CAD build for the part. Positions are in the model's coordinates, mm. A direction names the side the tool comes from. Round coordinates to 2 decimals unless told otherwise and drop trailing zeros. Order: outer loops, then holes, each group sorted by start corner. A loop starts at its lowest first (then second) coordinate and runs counter-clockwise, first axis right, second up. Notation, with made-up numbers: M 11.25,14 L 21.25,14 A37 cw 21.25,50 Z; hole C 48,68 d5. An arc over 180 degrees is marked long. Put each result on its own line as item: value.
```python
from build123d import *

# Parameters (mm, degrees)
SKETCH1_W                = 9
SKETCH1_H                = 2
BOSS_EXTRUDE1_DEPTH      = 15
CUT_EXTRUDE1_START       = -31
SKETCH2_W                = 8
SKETCH2_H                = 0.6
CUT_EXTRUDE1_DEPTH       = 32
SKETCH3_W                = 7.634272068
SKETCH3_H                = 0.75
CUT_EXTRUDE2_DEPTH       = 0.2
LPATTERN1_COUNT          = 19
LPATTERN1_PITCH          = 1.5
MIRROR2_COPY_1_SKETCH_W  = 7.634272068
MIRROR2_COPY_1_SKETCH_H  = 0.75
MIRROR2_COPY_1_DEPTH     = 0.2
MIRROR2_COPY_2_SKETCH_W  = 7.634272068
MIRROR2_COPY_2_SKETCH_H  = 0.75
MIRROR2_COPY_2_DEPTH     = 0.2
MIRROR2_COPY_3_SKETCH_W  = 7.634272068
MIRROR2_COPY_3_SKETCH_H  = 0.75
MIRROR2_COPY_3_DEPTH     = 0.2
MIRROR2_COPY_4_SKETCH_W  = 7.634272068
MIRROR2_COPY_4_SKETCH_H  = 0.75
MIRROR2_COPY_4_DEPTH     = 0.2
MIRROR2_COPY_5_SKETCH_W  = 7.634272068
MIRROR2_COPY_5_SKETCH_H  = 0.75
MIRROR2_COPY_5_DEPTH     = 0.2
MIRROR2_COPY_6_SKETCH_W  = 7.634272068
MIRROR2_COPY_6_SKETCH_H  = 0.75
MIRROR2_COPY_6_DEPTH     = 0.2
MIRROR2_COPY_7_SKETCH_W  = 7.634272068
MIRROR2_COPY_7_SKETCH_H  = 0.75
MIRROR2_COPY_7_DEPTH     = 0.2
MIRROR2_COPY_8_SKETCH_W  = 7.634272068
MIRROR2_COPY_8_SKETCH_H  = 0.75
MIRROR2_COPY_8_DEPTH     = 0.2
MIRROR2_COPY_9_SKETCH_W  = 7.634272068
MIRROR2_COPY_9_SKETCH_H  = 0.75
MIRROR2_COPY_9_DEPTH     = 0.2
MIRROR2_COPY_10_SKETCH_W = 7.634272068
MIRROR2_COPY_10_SKETCH_H = 0.75
MIRROR2_COPY_10_DEPTH    = 0.2
MIRROR2_COPY_11_SKETCH_W = 7.634272068
MIRROR2_COPY_11_SKETCH_H = 0.75
MIRROR2_COPY_11_DEPTH    = 0.2
MIRROR2_COPY_12_SKETCH_W = 7.634272068
MIRROR2_COPY_12_SKETCH_H = 0.75
MIRROR2_COPY_12_DEPTH    = 0.2
MIRROR2_COPY_13_SKETCH_W = 7.634272068
MIRROR2_COPY_13_SKETCH_H = 0.75
MIRROR2_COPY_13_DEPTH    = 0.2
MIRROR2_COPY_14_SKETCH_W = 7.634272068
MIRROR2_COPY_14_SKETCH_H = 0.75
MIRROR2_COPY_14_DEPTH    = 0.2
MIRROR2_COPY_15_SKETCH_W = 7.634272068
MIRROR2_COPY_15_SKETCH_H = 0.75
MIRROR2_COPY_15_DEPTH    = 0.2
MIRROR2_COPY_16_SKETCH_W = 7.634272068
MIRROR2_COPY_16_SKETCH_H = 0.75
MIRROR2_COPY_16_DEPTH    = 0.2
MIRROR2_COPY_17_SKETCH_W = 7.634272068
MIRROR2_COPY_17_SKETCH_H = 0.75
MIRROR2_COPY_17_DEPTH    = 0.2
MIRROR2_COPY_18_SKETCH_W = 7.634272068
MIRROR2_COPY_18_SKETCH_H = 0.75
MIRROR2_COPY_18_DEPTH    = 0.2


with BuildPart() as part:
    # Sketch1 → Boss-Extrude1 (new body, symmetric)
    with BuildSketch(Plane(origin=(0, 0, 0), x_dir=(1, 0, 0), z_dir=(0, 1, 0))):
        Rectangle(SKETCH1_W, SKETCH1_H)
    extrude(amount=BOSS_EXTRUDE1_DEPTH, both=True)

    # Sketch2 → Cut-Extrude1 (cut)
    with BuildSketch(Plane(origin=(0, 15, 0), x_dir=(1, 0, 0), z_dir=(0, 1, 0)).offset(CUT_EXTRUDE1_START)):
        with Locations((0, 0.5)):
            Rectangle(SKETCH2_W, SKETCH2_H)
    cut_extrude1 = extrude(amount=CUT_EXTRUDE1_DEPTH, mode=Mode.SUBTRACT)

    # Mirror1: Cut-Extrude1 across plane
    add(cut_extrude1.mirror(Plane.XY), mode=Mode.SUBTRACT)

    # Sketch3 → Cut-Extrude2 (cut)
    with BuildSketch(Plane.XY.offset(1)):
        with Locations((0, 13.875)):
            Rectangle(SKETCH3_W, SKETCH3_H)
    cut_extrude2 = extrude(amount=-CUT_EXTRUDE2_DEPTH, mode=Mode.SUBTRACT)

    # LPattern1: Cut-Extrude2 ×19
    with Locations(*[(0, -i * LPATTERN1_PITCH, 0) for i in range(1, LPATTERN1_COUNT)]):
        add(cut_extrude2, mode=Mode.SUBTRACT)

    # Mirror2: Cut-Extrude2 across plane
    add(cut_extrude2.mirror(Plane.XY), mode=Mode.SUBTRACT)

    # Mirror2 copy 1 sketch → Mirror2 copy 1 (cut)
    with BuildSketch(Plane(origin=(0, -1.5, -1), x_dir=(1, 0, 0), z_dir=(0, 0, -1))):
        with Locations((0, -13.875)):
            Rectangle(MIRROR2_COPY_1_SKETCH_W, MIRROR2_COPY_1_SKETCH_H)
    extrude(amount=-MIRROR2_COPY_1_DEPTH, mode=Mode.SUBTRACT)

    # Mirror2 copy 2 sketch → Mirror2 copy 2 (cut)
    with BuildSketch(Plane(origin=(0, -3, -1), x_dir=(1, 0, 0), z_dir=(0, 0, -1))):
        with Locations((0, -13.875)):
            Rectangle(MIRROR2_COPY_2_SKETCH_W, MIRROR2_COPY_2_SKETCH_H)
    extrude(amount=-MIRROR2_COPY_2_DEPTH, mode=Mode.SUBTRACT)

    # Mirror2 copy 3 sketch → Mirror2 copy 3 (cut)
    with BuildSketch(Plane(origin=(0, -4.5, -1), x_dir=(1, 0, 0), z_dir=(0, 0, -1))):
        with Locations((0, -13.875)):
            Rectangle(MIRROR2_COPY_3_SKETCH_W, MIRROR2_COPY_3_SKETCH_H)
    extrude(amount=-MIRROR2_COPY_3_DEPTH, mode=Mode.SUBTRACT)

    # Mirror2 copy 4 sketch → Mirror2 copy 4 (cut)
    with BuildSketch(Plane(origin=(0, -6, -1), x_dir=(1, 0, 0), z_dir=(0, 0, -1))):
        with Locations((0, -13.875)):
            Rectangle(MIRROR2_COPY_4_SKETCH_W, MIRROR2_COPY_4_SKETCH_H)
    extrude(amount=-MIRROR2_COPY_4_DEPTH, mode=Mode.SUBTRACT)

    # Mirror2 copy 5 sketch → Mirror2 copy 5 (cut)
    with BuildSketch(Plane(origin=(0, -7.5, -1), x_dir=(1, 0, 0), z_dir=(0, 0, -1))):
        with Locations((0, -13.875)):
            Rectangle(MIRROR2_COPY_5_SKETCH_W, MIRROR2_COPY_5_SKETCH_H)
    extrude(amount=-MIRROR2_COPY_5_DEPTH, mode=Mode.SUBTRACT)

    # Mirror2 copy 6 sketch → Mirror2 copy 6 (cut)
    with BuildSketch(Plane(origin=(0, -9, -1), x_dir=(1, 0, 0), z_dir=(0, 0, -1))):
        with Locations((0, -13.875)):
            Rectangle(MIRROR2_COPY_6_SKETCH_W, MIRROR2_COPY_6_SKETCH_H)
    extrude(amount=-MIRROR2_COPY_6_DEPTH, mode=Mode.SUBTRACT)

    # Mirror2 copy 7 sketch → Mirror2 copy 7 (cut)
    with BuildSketch(Plane(origin=(0, -10.5, -1), x_dir=(1, 0, 0), z_dir=(0, 0, -1))):
        with Locations((0, -13.875)):
            Rectangle(MIRROR2_COPY_7_SKETCH_W, MIRROR2_COPY_7_SKETCH_H)
    extrude(amount=-MIRROR2_COPY_7_DEPTH, mode=Mode.SUBTRACT)

    # Mirror2 copy 8 sketch → Mirror2 copy 8 (cut)
    with BuildSketch(Plane(origin=(0, -12, -1), x_dir=(1, 0, 0), z_dir=(0, 0, -1))):
        with Locations((0, -13.875)):
            Rectangle(MIRROR2_COPY_8_SKETCH_W, MIRROR2_COPY_8_SKETCH_H)
    extrude(amount=-MIRROR2_COPY_8_DEPTH, mode=Mode.SUBTRACT)

    # Mirror2 copy 9 sketch → Mirror2 copy 9 (cut)
    with BuildSketch(Plane(origin=(0, -13.5, -1), x_dir=(1, 0, 0), z_dir=(0, 0, -1))):
        with Locations((0, -13.875)):
            Rectangle(MIRROR2_COPY_9_SKETCH_W, MIRROR2_COPY_9_SKETCH_H)
    extrude(amount=-MIRROR2_COPY_9_DEPTH, mode=Mode.SUBTRACT)

    # Mirror2 copy 10 sketch → Mirror2 copy 10 (cut)
    with BuildSketch(Plane(origin=(0, -15, -1), x_dir=(1, 0, 0), z_dir=(0, 0, -1))):
        with Locations((0, -13.875)):
            Rectangle(MIRROR2_COPY_10_SKETCH_W, MIRROR2_COPY_10_SKETCH_H)
    extrude(amount=-MIRROR2_COPY_10_DEPTH, mode=Mode.SUBTRACT)

    # Mirror2 copy 11 sketch → Mirror2 copy 11 (cut)
    with BuildSketch(Plane(origin=(0, -16.5, -1), x_dir=(1, 0, 0), z_dir=(0, 0, -1))):
        with Locations((0, -13.875)):
            Rectangle(MIRROR2_COPY_11_SKETCH_W, MIRROR2_COPY_11_SKETCH_H)
    extrude(amount=-MIRROR2_COPY_11_DEPTH, mode=Mode.SUBTRACT)

    # Mirror2 copy 12 sketch → Mirror2 copy 12 (cut)
    with BuildSketch(Plane(origin=(0, -18, -1), x_dir=(1, 0, 0), z_dir=(0, 0, -1))):
        with Locations((0, -13.875)):
            Rectangle(MIRROR2_COPY_12_SKETCH_W, MIRROR2_COPY_12_SKETCH_H)
    extrude(amount=-MIRROR2_COPY_12_DEPTH, mode=Mode.SUBTRACT)

    # Mirror2 copy 13 sketch → Mirror2 copy 13 (cut)
    with BuildSketch(Plane(origin=(0, -19.5, -1), x_dir=(1, 0, 0), z_dir=(0, 0, -1))):
        with Locations((0, -13.875)):
            Rectangle(MIRROR2_COPY_13_SKETCH_W, MIRROR2_COPY_13_SKETCH_H)
    extrude(amount=-MIRROR2_COPY_13_DEPTH, mode=Mode.SUBTRACT)

    # Mirror2 copy 14 sketch → Mirror2 copy 14 (cut)
    with BuildSketch(Plane(origin=(0, -21, -1), x_dir=(1, 0, 0), z_dir=(0, 0, -1))):
        with Locations((0, -13.875)):
            Rectangle(MIRROR2_COPY_14_SKETCH_W, MIRROR2_COPY_14_SKETCH_H)
    extrude(amount=-MIRROR2_COPY_14_DEPTH, mode=Mode.SUBTRACT)

    # Mirror2 copy 15 sketch → Mirror2 copy 15 (cut)
    with BuildSketch(Plane(origin=(0, -22.5, -1), x_dir=(1, 0, 0), z_dir=(0, 0, -1))):
        with Locations((0, -13.875)):
            Rectangle(MIRROR2_COPY_15_SKETCH_W, MIRROR2_COPY_15_SKETCH_H)
    extrude(amount=-MIRROR2_COPY_15_DEPTH, mode=Mode.SUBTRACT)

    # Mirror2 copy 16 sketch → Mirror2 copy 16 (cut)
    with BuildSketch(Plane(origin=(0, -24, -1), x_dir=(1, 0, 0), z_dir=(0, 0, -1))):
        with Locations((0, -13.875)):
            Rectangle(MIRROR2_COPY_16_SKETCH_W, MIRROR2_COPY_16_SKETCH_H)
    extrude(amount=-MIRROR2_COPY_16_DEPTH, mode=Mode.SUBTRACT)

    # Mirror2 copy 17 sketch → Mirror2 copy 17 (cut)
    with BuildSketch(Plane(origin=(0, -25.5, -1), x_dir=(1, 0, 0), z_dir=(0, 0, -1))):
        with Locations((0, -13.875)):
            Rectangle(MIRROR2_COPY_17_SKETCH_W, MIRROR2_COPY_17_SKETCH_H)
    extrude(amount=-MIRROR2_COPY_17_DEPTH, mode=Mode.SUBTRACT)

    # Mirror2 copy 18 sketch → Mirror2 copy 18 (cut)
    with BuildSketch(Plane(origin=(0, -27, -1), x_dir=(1, 0, 0), z_dir=(0, 0, -1))):
        with Locations((0, -13.875)):
            Rectangle(MIRROR2_COPY_18_SKETCH_W, MIRROR2_COPY_18_SKETCH_H)
    extrude(amount=-MIRROR2_COPY_18_DEPTH, mode=Mode.SUBTRACT)


solid = part.part
```
Item 1: Band-saw the part on B-B on x = 0. State how many separate pieces and enclosed holes the cut face has, and give its area (3 significant figures).
Answers below:
separate pieces: 41
enclosed holes: 0
area: 18.3 mm²
Item 2: Mould opens along Z. For faces 1 (the flat face through (-0.1, -0.2, -0.8)), 2 (the flat face through (-4, 0, 1)), 3 (the flat face through (-4.5, 0, 0)), 4 (the flat face through (0, 0, 0.2)) say: pulls with the +Z half, pulls with the -Z half, needs draft (parallel to the pull), parting line crosses it, or undercut.
Answers below:
face 1: undercut
face 2: pulls with the +Z half
face 3: needs draft
face 4: undercut
Item 3: Probe line 1 along Z through (x, y) = (-1.25, 4); line 2 along X through (y, z) = (-13, 0.25); line 3 along Z through (x, y) = (0, 9.5). List the from-to ranges inside material, lowest first. Write a range as [from, to].
Answers below:
line 1: [-1, -0.8], [-0.2, 0.2], [0.8, 1]
line 2: [-4.5, -4], [4, 4.5]
line 3: [-0.2, 0.2]
Item 4: Band-saw the part on A-A on z = -0.5. Give the cut face in (x, y).
Answers below:
outline: M -4.5,-15 L -4,-15 L -4,15 L -4.5,15 Z; M 4,-15 L 4.5,-15 L 4.5,15 L 4,15 Z
Item 5: Pin check, flat tip, straight feed: P1, Ø1, axis at x = -2.5, z = 0.5, coming from the -Y side. Stop position of the tip, or through.
Answers below:
P1: y = -15
Item 6: Tool access for faces 5 (the flat face through (0, 0, -0.2)), 6 (the flat face through (-1, 15, 0)): list every direction of +Z, -Z, +X, -X, +Y, -Y with a clear straight run to the whole face (end or side of a thin tool).
Answers below:
face 5: +Y, -Y
face 6: +Z, -Z, +X, -X, +Y
